```python
from build123d import *

# Parameters (mm, degrees)
F0_R     = 15
F1_DEPTH = 10
F2_R     = 10
F3_DEPTH = 48
F4_SIZE  = 1


with BuildPart() as f1:
    # F0 (on Front) → F1 (new body)
    with BuildSketch(Plane.XZ):
        Circle(F0_R)
    extrude(amount=-F1_DEPTH)

    # F2 (on face) → F3 (join)
    with BuildSketch(Plane(origin=(0, 10, 0), x_dir=(-1, 0, 0), z_dir=(0, 1, 0))):
        Circle(F2_R)
    extrude(amount=F3_DEPTH)

    # F4
    f4_edges = [f1.edges().sort_by_distance(p)[0] for p in [
        (10, 58, 0),
        (-15, 0, 0),
    ]]
    chamfer(f4_edges, length=F4_SIZE)


solid = f1.part
```
CAD build for the part. Positions are in the model's coordinates, mm. A direction names the side the tool comes from. Round coordinates to 2 decimals unless told otherwise and drop trailing zeros. Write each loop counter-clockwise with the first axis right and the second up, starting at its lowest first coordinate (ties: lowest second). Pieces come first, ordered by that corner, then holes.
Item 1: Drill centre lines: L1, parallel to Y at x = 2.25, z = -10.75; L2, parallel to X at y = 43, z = 0.5. Where is each one in solid material? Low to high.
Filled in:
L1: y = 0 to 10
L2: x = -9.99 to 9.99
Item 2: Band-saw the part on C-C on y = 22.5. Write the cut outline in (x, z).
Filled in:
outline: circle Ø20 at (0, 0)
Item 3: Band-saw the part on A-A on z = 0. Write the cut outline in (x, y), then the cut area to 3 significant figures.
Filled in:
outline: (-15, 1) - (-14, 0) - (14, 0) - (15, 1) - (15, 10) - (10, 10) - (10, 57) - (9, 58) - (-9, 58) - (-10, 57) - (-10, 10) - (-15, 10) - close
area: 1,260 mm2
Item 4: Band-saw the part on B-B on x = 0. Write the cut outline in (y, z), then the cut area to 3 significant figures.
Filled in:
outline: (0, -14) - (1, -15) - (10, -15) - (10, -10) - (57, -10) - (58, -9) - (58, 9) - (57, 10) - (10, 10) - (10, 15) - (1, 15) - (0, 14) - close
area: 1,260 mm2
Item 5: Drop flat-ended pins along their axis: pin 1 Ø12 at (x, y) = (7, 11.5) entering from -Z; pin 2 Ø5 at (y, z) = (15.5, 4) entering from -X; pin 3 Ø1.5 at (y, z) = (8, 10.5) entering from -X; pin 4 Ø6 at (x, z) = (7, -2) entering from -Y. Give the stop position or say it passes through.
Filled in:
pin 1: stops at z = -14.95
pin 2: stops at x = -9.89
pin 3: stops at x = -11.4
pin 4: stops at y = 0
Item 6: Tool access for faces 1 (the flat face through (0, 0, 0)), 2 (the cylindrical face through (2.17, 33.17, -9.76)): list every direction of +Z, -Z, +X, -X, +Y, -Y with a clear straight run to the whole face (end or side of a thin tool).
Filled in:
face 1: +Z, -Z, +X, -X, -Y
face 2: +Y
